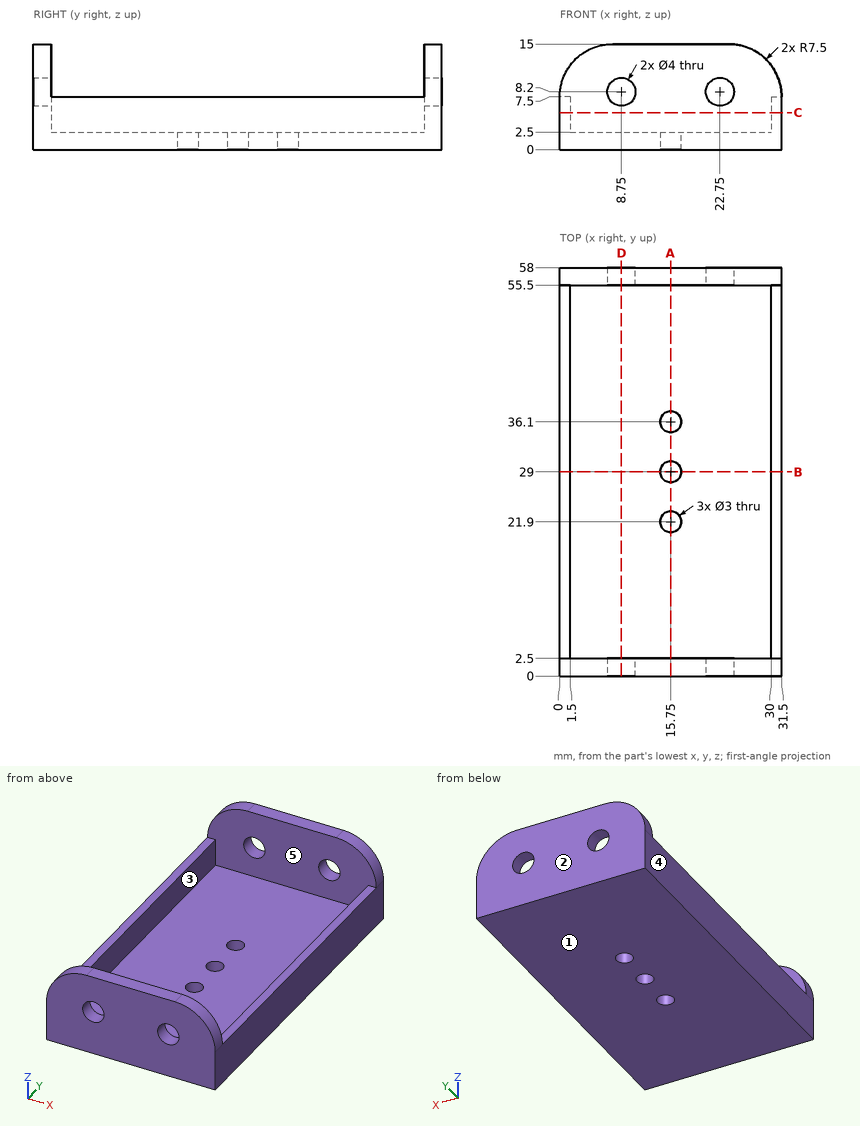
Verification items for this drawing (mm, ordinates from the low corner). A direction names the side the tool comes from. Give positions to 0.01 mm unless a question says otherwise; leave off trailing zeros. Loops run counter-clockwise (first coordinate to the right, second up) from the corner with the lowest first, then second, coordinate; pieces in that order, holes last.
(1) Section check D-D on x = 8.75. Record the cut outline in (y, z).
From the geometry:
outline: (0, 0) - (58, 0) - (58, 6.2) - (55.5, 6.2) - (55.5, 2.5) - (2.5, 2.5) - (2.5, 6.2) - (0, 6.2) - close; (0, 10.2) - (2.5, 10.2) - (2.5, 15) - (0, 15) - close; (55.5, 10.2) - (58, 10.2) - (58, 15) - (55.5, 15) - close
(2) Thickness scan on L1, parallel to Y at x = 15.75, z = 1.4; L2, parallel to X at y = 27, z = 3.5; L3, parallel to X at y = 29, z = 0.95. Record the ranges inside material, lowest first.
From the geometry:
L1: y = 0 to 20.4, 23.4 to 27.5, 30.5 to 34.6, 37.6 to 58
L2: x = 0 to 1.5, 30 to 31.5
L3: x = 0 to 14.25, 17.25 to 31.5
(3) Section check B-B on y = 29. Record the cut outline in (x, z), then the cut area to 4 significant figures.
From the geometry:
outline: (0, 0) - (14.25, 0) - (14.25, 2.5) - (1.5, 2.5) - (1.5, 7.5) - (0, 7.5) - close; (17.25, 0) - (31.5, 0) - (31.5, 7.5) - (30, 7.5) - (30, 2.5) - (17.25, 2.5) - close
area: 86.25 mm2
(4) Release check for a two-part mould opening along Y. For the marked faces 1, 2 and 3 record: released by +Y, released by -Y, zero draft, split by the parting line, or undercut.
From the geometry:
face 1: zero draft
face 2: released by +Y
face 3: undercut
(5) Section check A-A on x = 15.75. Record the cut outline in (y, z), then the cut area to 3 significant figures.
From the geometry:
outline: (0, 0) - (20.4, 0) - (20.4, 2.5) - (2.5, 2.5) - (2.5, 15) - (0, 15) - close; (23.4, 0) - (27.5, 0) - (27.5, 2.5) - (23.4, 2.5) - close; (30.5, 0) - (34.6, 0) - (34.6, 2.5) - (30.5, 2.5) - close; (37.6, 0) - (58, 0) - (58, 15) - (55.5, 15) - (55.5, 2.5) - (37.6, 2.5) - close
area: 185 mm2
(6) Depth check by flat-ended pin: pin 1 Ø0.5 at (x, y) = (30.5, 38) entering from +Z; pin 2 Ø3 at (x, z) = (26, 7.5) entering from -Y; pin 3 Ø1.5 at (x, y) = (20, 30.5) entering from +Z. Enter the tip coordinate at first touch or a pass-through.
From the geometry:
pin 1: stops at z = 7.5
pin 2: stops at y = 0
pin 3: stops at z = 2.5
(7) Section check C-C on z = 5.25. Record the cut outline in (x, y).
From the geometry:
outline: (0, 0) - (31.5, 0) - (31.5, 58) - (0, 58) - close; hole (1.5, 2.5) - (30, 2.5) - (30, 55.5) - (1.5, 55.5) - close
(8) Set-up check for the marked faces 4 and 5: record each of +Z, -Z, +X, -X, +Y, -Y from which the full face is reachable in a straight line by a thin tool's end or side.
From the geometry:
face 4: +Z, -Z, -X, +Y, -Y
face 5: +Z
